```python
from build123d import *

# Parameters (mm, degrees)
SKETCH_1_R          = 4
EXTRUDE_1_DEPTH     = 17.1
SKETCH_2_R          = 5
EXTRUDE_2_DEPTH     = 102
SKETCH_3_R          = 1.65
CUT_EXTRUDE_1_DEPTH = 20
CUT_EXTRUDE_START   = -6.8
SKETCH_7_R          = 5
SKETCH_7_R_2        = 3.95
CUT_EXTRUDE_4_DEPTH = 1.1
SKETCH_8_R          = 3
EXTRUDE_3_DEPTH     = 2.5
CHAMFER_1_SIZE      = 0.5
SKETCH_9_R          = 1.25
CUT_EXTRUDE_5_DEPTH = 7
CUT_EXTRUDE_START_2 = -10
SKETCH_7_2_R        = 5
SKETCH_7_2_R_2      = 3.95
CUT_EXTRUDE_6_DEPTH = 1.1


with BuildPart() as part:
    # 草图1 → 凸台-拉伸1 (new body)
    with BuildSketch(Plane(origin=(0, 0, 0), x_dir=(0, 0, -1), z_dir=(1, 0, 0))):
        Circle(SKETCH_1_R)
    extrude(amount=EXTRUDE_1_DEPTH)

    # 草图2 → 凸台-拉伸2 (add)
    with BuildSketch(Plane(origin=(17.1, 0, 0), x_dir=(0, 0, -1), z_dir=(1, 0, 0))):
        with Locations(Location((0, 0, 0), (0, 0, 270))):
            Circle(SKETCH_2_R)
    extrude(amount=EXTRUDE_2_DEPTH)

    # 草图3 → 切除-拉伸1 (cut)
    with BuildSketch(Plane(origin=(0, 7, 0), x_dir=(1, 0, 0), z_dir=(0, 1, 0))):
        with Locations(Location((3.5, 0, 0), (0, 0, 270))):
            Circle(SKETCH_3_R)
    extrude(amount=-CUT_EXTRUDE_1_DEPTH, mode=Mode.SUBTRACT)

    # 草图7 → 切除-拉伸4 (cut)
    with BuildSketch(Plane.ZY.offset(-97.6).offset(CUT_EXTRUDE_START)):
        Circle(SKETCH_7_R)
        Circle(SKETCH_7_R_2, mode=Mode.SUBTRACT)
    extrude(amount=-CUT_EXTRUDE_4_DEPTH, mode=Mode.SUBTRACT)

    # 草图8 → 凸台-拉伸3 (add)
    with BuildSketch(Plane(origin=(119.1, 0, 0), x_dir=(0, 0, -1), z_dir=(1, 0, 0))):
        Circle(SKETCH_8_R)
    extrude(amount=EXTRUDE_3_DEPTH)

    # 倒角1
    chamfer_1_edges = [part.edges().sort_by_distance(p)[0] for p in [
        (0, 0, 4),
        (121.6, 0, 3),
    ]]
    chamfer(chamfer_1_edges, length=CHAMFER_1_SIZE)

    # 草图9 → 切除-拉伸5 (cut)
    with BuildSketch(Plane(origin=(0, 5, 0), x_dir=(1, 0, 0), z_dir=(0, 1, 0))):
        with Locations(Location((83.1, 0, 0), (0, 0, 270))):
            Circle(SKETCH_9_R)
        with Locations(Location((55.1, 0, 0), (0, 0, 270))):
            Circle(SKETCH_9_R)
    extrude(amount=-CUT_EXTRUDE_5_DEPTH, mode=Mode.SUBTRACT)

    # 草图7<2> → 切除-拉伸6 (cut)
    with BuildSketch(Plane.ZY.offset(-97.6).offset(CUT_EXTRUDE_START_2)):
        Circle(SKETCH_7_2_R)
        Circle(SKETCH_7_2_R_2, mode=Mode.SUBTRACT)
    extrude(amount=-CUT_EXTRUDE_6_DEPTH, mode=Mode.SUBTRACT)


solid = part.part
```
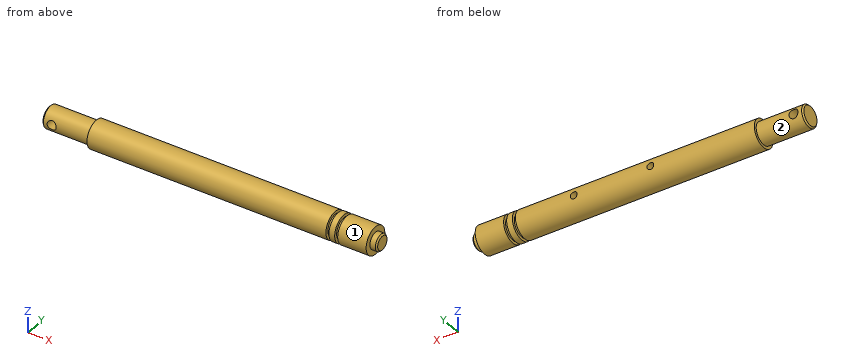
Model file for the job. Use its own axes, mm. Face numbers are marked on the shaded views. A direction names the side the tool comes from. Coordinates: 2 decimals unless noted, no trailing zeros. Loops run counter-clockwise (first coordinate to the right, second up) from the corner with the lowest first, then second, coordinate; pieces in that order, holes last. Notation, with made-up numbers: M -32.5,24 L 10.5,24 A6 cw 10.5,33 Z; hole C 54,6.5 d3. An arc over 180 degrees is marked long. Use CSV: the item, a comma, the result in double quotes. Start each with the question number.
1. Band-saw the part on A-A, the plane y = 0. Give the number of separate pieces and of enclosed holes in the cut face, then the cut area to 3 significant figures.
2. Flat gauge pins, fed straight in: pin 1 (1.2 mm diameter, centred on x = 55.5, z = 0, fed in from +Y); pin 2 (1.5 mm diameter, centred on x = 48, z = 1.5, fed in from -Y); pin 3 (1 mm diameter, centred on x = 81, z = -1, fed in from -Y). Where does each tip first touch, or does it go through?
3. Band-saw the part on D-D, the plane x = 55.1. List the corners of the cut face in (y, z), then the cut area to 3 significant figures.
4. Tool access for the marked faces 1 and 2: list every direction of +Z, -Z, +X, -X, +Y, -Y with a clear straight run to the whole face (end or side of a thin tool).
5. Band-saw the part on B-B, the plane x = 95.5. List the corners of the cut face in (y, z), then the cut area to 3 significant figures.
6. Probe probe 1 along X at (y, z) = (1.75, 3.75); probe 2 along X at (y, z) = (-0.5, 0); probe 3 along Z at (x, y) = (55.1, -0.5). List the from-to ranges inside material, lowest first. Write a range as [from, to].
7. Band-saw the part on C-C, the plane x = 3.5. List the corners of the cut face in (y, z), then the cut area to 3 significant figures.
Entries:
1,separate pieces,"1"
1,enclosed holes,"3"
1,area,"1,150 mm2"
2,pin 1,"stops at y = -2"
2,pin 2,"stops at y = -4.94"
2,pin 3,"stops at y = -4.97"
3,outline,"M -2,-1.25 L -2,1.25 L 4.84,1.25 A5 ccw long 4.84,-1.25 Z"
3,area,"61.2 mm2"
4,face 1,"+X, -X"
4,face 2,"-X"
5,outline,"C 0,0 d10"
5,area,"78.5 mm2"
6,probe 1,"x = [17.1, 104.4], [105.5, 107.6], [108.7, 119.1]"
6,probe 2,"x = [0, 1.85], [5.15, 53.85], [56.35, 81.85], [84.35, 121.6]"
6,probe 3,"z = [-4.97, -1.25], [1.25, 4.97]"
7,outline,"M -3.64,-1.65 A4 ccw 3.64,-1.65 Z; M -3.64,1.65 L 3.64,1.65 A4 ccw Z"
7,area,"24.6 mm2"
